```python
from build123d import *

# Parameters (mm, degrees)
F0_R      = 17.3609
F1_DEPTH  = 24.384
F2_R      = 14.986
F3_DEPTH  = 49.0982
F4_R      = 1.016
F5_DEPTH  = 6.35
F6_R      = 6.35
F6_R_2    = 3.175
F7_DEPTH  = 1.5875
F8_R      = 1.9812
F9_DEPTH  = 2.8448
F10_R     = 1.2065
F11_DEPTH = 6.35
F12_R     = 6.35
F12_R_2   = 4.1275
F13_DEPTH = 1.3716
F14_R     = 2.38125
F15_DEPTH = 15.875


with BuildPart() as f1:
    # F0 (on Right) → F1 (new body)
    with BuildSketch(Plane.YZ):
        Circle(F0_R)
    extrude(amount=F1_DEPTH)

    # F2 (on face) → F3 (join)
    with BuildSketch(Plane.YZ.offset(24.384)):
        Circle(F2_R)
    extrude(amount=F3_DEPTH)

    # F4 (on face) → F5 (cut)
    with BuildSketch(Plane.YZ.offset(73.4822)):
        with Locations((0, 11.01725)):
            Circle(F4_R)
        with Locations((9.525, -5.480534)):
            Circle(F4_R)
        with Locations((-9.525, -5.480534)):
            Circle(F4_R)
    extrude(amount=-F5_DEPTH, mode=Mode.SUBTRACT)

    # F6 (on face) → F7 (join)
    with BuildSketch(Plane.YZ.offset(73.4822)):
        Circle(F6_R)
        Circle(F6_R_2, mode=Mode.SUBTRACT)
    extrude(amount=F7_DEPTH)

    # F8 (on face) → F9 (join)
    with BuildSketch(Plane.YZ.offset(73.4822)):
        Circle(F8_R)
    extrude(amount=F9_DEPTH)

    # F10 (on face) → F11 (cut)
    with BuildSketch(Plane(origin=(0, 0, 0), x_dir=(0, -1, 0), z_dir=(-1, 0, 0))):
        with Locations((0, 13.4239)):
            Circle(F10_R)
        with Locations((11.5951, -6.659402)):
            Circle(F10_R)
        with Locations((-11.5951, -6.659402)):
            Circle(F10_R)
    extrude(amount=-F11_DEPTH, mode=Mode.SUBTRACT)

    # F12 (on face) → F13 (join)
    with BuildSketch(Plane(origin=(0, 0, 0), x_dir=(0, -1, 0), z_dir=(-1, 0, 0))):
        with Locations((-1.7145, -6.4643)):
            Circle(F12_R)
        with Locations((-1.7145, -6.4643)):
            Circle(F12_R_2, mode=Mode.SUBTRACT)
    extrude(amount=F13_DEPTH)

    # F14 (on face) → F15 (join)
    with BuildSketch(Plane(origin=(0, 0, 0), x_dir=(0, -1, 0), z_dir=(-1, 0, 0))):
        with Locations((-1.7145, -6.4643)):
            Circle(F14_R)
    extrude(amount=F15_DEPTH)


solid = f1.part
```
Work out the finished part from the listing and answer in its coordinate system (mm). A direction names the side the tool comes from. Round coordinates to 2 decimals unless told otherwise and drop trailing zeros. Loops run counter-clockwise (first coordinate to the right, second up) from the corner with the lowest first, then second, coordinate; pieces in that order, holes last. Notation, with made-up numbers: M -8,64.5 L 43,64.5 A22 ccw 43,82.5 Z; hole C -35,-1 d6. An arc over 180 degrees is marked long. One line per question, with ' | ' between items.
Q1. Each of these flat-tipped pins is pushed along its axis until it touches: pin 1 Ø1 at (y, z) = (-10, -5.5) entering from +X; pin 2 Ø1.9 at (y, z) = (11.6, -6.66) entering from -X; pin 3 Ø1.6 at (y, z) = (-9.52, -5.48) entering from -X. Where does it stop, or does it pass through?
Conclusion:
pin 1: stops at x = 67.13 | pin 2: stops at x = 6.35 | pin 3: stops at x = 0
Q2. The mould has two halves that part along Y. Classify faces 1 (the flat face through (0, 0, 0)), 2 (the cylindrical face through (74.885, -0.258, 1.964)), 3 (the cylindrical face through (-0.68, 2.54, -0.17)): +Y half, -Y half, draft (parallel to the pull), parting line (faces both ways), or undercut.
Conclusion:
face 1: draft | face 2: undercut | face 3: parting line
Q3. Consider line 1 along X through (y, z) = (-16, 1); line 2 along X through (y, z) = (-4.5, -2.5); line 3 along Z through (x, y) = (2, 0). Determine where each line is inside the solid, lowest interval first. Write a range as from..to.
Conclusion:
line 1: x = 0..24.38 | line 2: x = 0..75.07 | line 3: z = -17.36..12.22, 14.63..17.36
Q4. A tool of negligible diameter and unlimited length cuts with its end or side. For faces 4 (the cylindrical face through (3.13, -0.65, 14.44)), 5 (the flat face through (73.482, -0.2, -6.5)), 6 (the flat face through (76.327, 0, 0)), from which of +Z, -Z, +X, -X, +Y, -Y can it reach the whole face along a straight path? Write none if from no direction.
Conclusion:
face 4: -X | face 5: +X | face 6: +Z, -Z, +X, +Y, -Y
Q5. Find section C-C, the plane x = -2.5. Give the vertices of the cut face in (y, z), then the cut area to 3 significant figures.
Conclusion:
outline: C 1.71,-6.46 d4.76 | area: 17.8 mm2
Q6. Find section B-B, the plane x = 55.5. Give the vertices of the cut face in (y, z), then the cut area to 3 significant figures.
Conclusion:
outline: C 0,0 d29.97 | area: 706 mm2
Q7. Find section A-A, the plane z = -14. Give the vertices of the cut face in (x, y).
Conclusion:
outline: M 0,-10.27 L 24.38,-10.27 L 24.38,-5.35 L 73.48,-5.35 L 73.48,5.35 L 24.38,5.35 L 24.38,10.27 L 0,10.27 Z
